Part model, mm, in its own coordinate system. A direction names the side the tool comes from. Give positions to 0.01 mm unless a question says otherwise; leave off trailing zeros. Loops run counter-clockwise (first coordinate to the right, second up) from the corner with the lowest first, then second, coordinate; pieces in that order, holes last. Notation, with made-up numbers: (32.5, -14.75) -> (70.5, -14.75) arc R31 ccw to (70.5, 17.25) -> close; hole circle Ø1 at (-26, -22.5). An arc over 180 degrees is marked (long way). One line per question, with ' | ' between items.
```python
from build123d import *

# Parameters (mm, degrees)
SKETCH1_R            = 75
SKETCH1_R_2          = 70
BOSS_EXTRUDE1_DEPTH  = 140
SKETCH2_W            = 20
SKETCH2_H            = 130
BOSS_EXTRUDE2_DEPTH  = 10
FILLET1_R            = 9
FILLET2_R            = 10
FILLET3_R            = 5
SKETCH5_W            = 4
SKETCH5_H            = 19
CUT_EXTRUDE1_DEPTH   = 10
FILLET4_R            = 2
FILLET4_OF_MIRROR4_R = 2


# Some blends are built 0.0001 mm under size
with BuildPart() as part:
    # Sketch1 → Boss-Extrude1 (new body)
    with BuildSketch(Plane(origin=(0, 0, 0), x_dir=(1, 0, 0), z_dir=(0, 1, 0))):
        with Locations(Location((0, 0, 0), (0, 0, 270))):
            Circle(SKETCH1_R)
        with Locations(Location((0, 0, 0), (0, 0, 270))):
            Circle(SKETCH1_R_2, mode=Mode.SUBTRACT)
    extrude(amount=BOSS_EXTRUDE1_DEPTH)

    # Sketch2 → Boss-Extrude2 (add)
    with BuildSketch(Plane(origin=(0, 140, 0), x_dir=(1, 0, 0), z_dir=(0, 1, 0))):
        with Locations((-65, 0)):
            Rectangle(SKETCH2_W, SKETCH2_H)
    extrude(amount=BOSS_EXTRUDE2_DEPTH)

    # Fillet1
    # the kernel refuses this fillet: 9 mm, written as the material it adds along each edge
    with BuildSketch(Plane(origin=(0, 140, 0), x_dir=(-0.5499699922766536, 0, -0.835184415321082), z_dir=(0.835184415321082, 0, -0.5499699922766536))) as fillet1_piece_1_section:
        with BuildLine():
            CenterArc((70 - FILLET1_R, -FILLET1_R), FILLET1_R, 0, 90)
            Line((70 - FILLET1_R, 0), (70, 0))
            Line((70, 0), (70, -FILLET1_R))
        make_face()
    fillet1_piece_1 = revolve(axis=Axis((0, 140, 0), (0, 1, 0)), revolution_arc=113.270091323, mode=Mode.PRIVATE)
    fillet1_piece_1 = split(fillet1_piece_1, bisect_by=Plane(origin=(-55, 137.444603365, 0), z_dir=(-1, 0, 0)), keep=Keep.TOP, mode=Mode.PRIVATE)
    add(fillet1_piece_1)

    # Fillet2
    # the kernel refuses this fillet: 10 mm, written as the material it adds along each edge
    with BuildSketch(Plane(origin=(-55, 140, -75.990195136), x_dir=(0, 1, 0), z_dir=(0, 0, 1))) as fillet2_piece_1_section:
        with BuildLine():
            CenterArc((FILLET2_R, -FILLET2_R), FILLET2_R, 90, 90)
            Line((0, -FILLET2_R), (0, 0))
            Line((0, 0), (FILLET2_R, 0))
        make_face()
    fillet2_piece_1 = extrude(amount=57.688924947, mode=Mode.PRIVATE)
    fillet2_piece_1 = fillet2_piece_1 - Plane(origin=(0, 142.276585478, 0), x_dir=(0, 0, 1), z_dir=(0, -1, 0)) * Cylinder(70, 156, mode=Mode.PRIVATE)
    fillet2_piece_1 = fillet2_piece_1 & Plane(origin=(0, 142.276585478, 0), x_dir=(0, 0, 1), z_dir=(0, -1, 0)) * Cylinder(75, 156, mode=Mode.PRIVATE)
    add(fillet2_piece_1)
    with BuildSketch(Plane(origin=(-55, 140, 18.301270189), x_dir=(0, 1, 0), z_dir=(0, 0, 1))) as fillet2_piece_2_section:
        with BuildLine():
            CenterArc((FILLET2_R, -FILLET2_R), FILLET2_R, 90, 90)
            Line((0, -FILLET2_R), (0, 0))
            Line((0, 0), (FILLET2_R, 0))
        make_face()
    fillet2_piece_2 = extrude(amount=57.688924947, mode=Mode.PRIVATE)
    fillet2_piece_2 = fillet2_piece_2 - Plane(origin=(0, 142.276601392, 0), x_dir=(0, 0, 1), z_dir=(0, -1, 0)) * Cylinder(70, 156, mode=Mode.PRIVATE)
    fillet2_piece_2 = fillet2_piece_2 & Plane(origin=(0, 142.276601392, 0), x_dir=(0, 0, 1), z_dir=(0, -1, 0)) * Cylinder(75, 156, mode=Mode.PRIVATE)
    add(fillet2_piece_2)

    # Fillet3
    fillet3_edges = [part.edges().sort_by_distance(p)[0] for p in [
        (-75, 145, -65),
        (-75, 145, 65),
        (-55, 145, 65),
        (-55, 145, -65),
    ]]
    fillet(fillet3_edges, radius=FILLET3_R)

    # Sketch5 → Cut-Extrude1 (cut)
    with BuildSketch(Plane(origin=(0, 150, 0), x_dir=(1, 0, 0), z_dir=(0, 1, 0))):
        with Locations((-65, -51.5)):
            Rectangle(SKETCH5_W, SKETCH5_H)
    cut_extrude1 = extrude(amount=-CUT_EXTRUDE1_DEPTH, mode=Mode.SUBTRACT)

    # Fillet4
    fillet4_edges = [part.edges().sort_by_distance(p)[0] for p in [
        (-67, 145, 42),
        (-63, 145, 42),
        (-67, 145, 61),
        (-63, 145, 61),
    ]]
    fillet(fillet4_edges, radius=FILLET4_R - 0.0001)  # a hair under: the kernel refuses the full size

    # Mirror4: Cut-Extrude1 across plane
    add(cut_extrude1.mirror(Plane.XY), mode=Mode.SUBTRACT)

    # Fillet4 of Mirror4
    fillet4_of_mirror4_edges = [part.edges().sort_by_distance(p)[0] for p in [
        (-67, 145, -42),
        (-63, 145, -42),
        (-67, 145, -61),
        (-63, 145, -61),
    ]]
    fillet(fillet4_of_mirror4_edges, radius=FILLET4_OF_MIRROR4_R - 0.0001)  # a hair under: the kernel refuses the full size


solid = part.part
```
1) Saw through at C-C (x = -51.5). Give the cut face in (y, z).
Found:
outline: (0, -54.52) -> (142.4, -54.52) -> (142.4, -47.41) -> (0, -47.41) -> close; (0, 47.41) -> (142.4, 47.41) -> (142.4, 54.52) -> (0, 54.52) -> close
2) Saw through at A-A (x = 0). Give the cut face in (y, z), and give its area (3 significant figures).
Found:
outline: (0, -75) -> (140, -75) -> (140, -70) -> (0, -70) -> close; (0, 70) -> (140, 70) -> (140, 75) -> (0, 75) -> close | area: 1,400 mm2
3) Pin check, flat tips, straight feed: P1, Ø5, axis at y = 146.5, z = -49.5, coming from the +X side; P2, Ø10, axis at x = -18, y = 21, coming from the -Z side; P3, Ø4.5, axis at y = 146, z = 56.5, coming from the +X side. Stop position of each tip, or through.
Found:
P1: x = -53 | P2: z = -73.86 | P3: x = -55
4) Pull direction Z, two halves, no side cores. Call faces 1 (the flat face through (-75, 145, 1)), 2 (the cylindrical face through (-56, 145, 63)), 3 (the cylindrical face through (-56, 145, -63)), 4 (the flat face through (-63, 145, 52)): pulls with the +Z half, pulls with the -Z half, needs draft (parallel to the pull), parting line crosses it, or undercut.
Found:
face 1: needs draft | face 2: pulls with the +Z half | face 3: pulls with the -Z half | face 4: undercut
5) Drill centre lines: line 1 (X direction, y = 103, z = 0); line 2 (Y direction, x = -32.5, z = -65.5). Where is each one in solid material? Low to high.
Found:
line 1: -75 to -70, 70 to 75 | line 2: 0 to 140
6) Saw through at B-B (y = 85). Give the cut face in (x, z), and give its area (3 significant figures).
Found:
outline: circle Ø150 at (0, 0); hole circle Ø140 at (0, 0) | area: 2,280 mm2
7) Tool access for faces 5 (the flat face through (69, 140, -17)), 6 (the flat face through (-67.4, 140, -47.4)), 7 (the flat face through (-67.4, 140, 46.5)): list every direction of +Z, -Z, +X, -X, +Y, -Y with a clear straight run to the whole face (end or side of a thin tool).
Found:
face 5: +Z, -Z, +X, +Y | face 6: -Z, -X, -Y | face 7: +Z, -X, -Y
